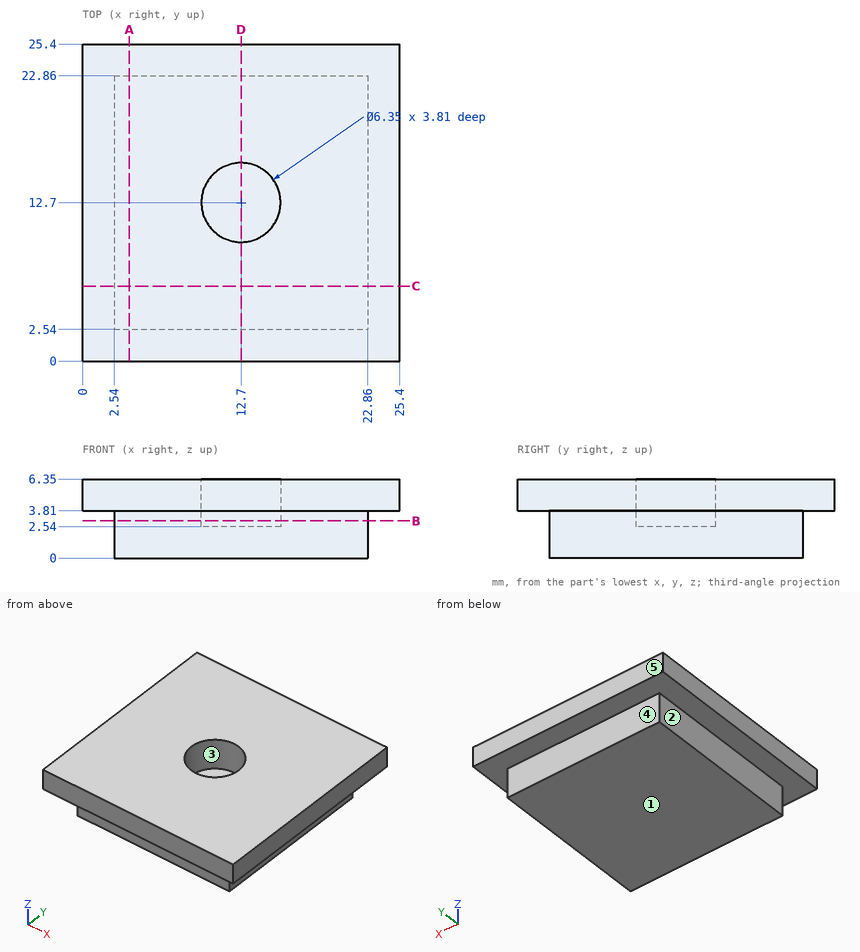
Source: three-view drawing plus pictorial views. Frame: mm from the lowest corner of the part. A direction names the side the tool comes from. Round coordinates to 2 decimals unless told otherwise and drop trailing zeros. Order: outer loops, then holes, each group sorted by start corner. A loop starts at its lowest first (then second) coordinate and runs counter-clockwise, first axis right, second up. Notation, with made-up numbers: (13.5, 30.25) - (23.5, 30.25) arc R36 cw to (23.5, 65.25) - close; hole circle Ø11 at (-35, -36.75). An arc over 180 degrees is marked (long way). Write each question's results on one line, items separated by ' | '.
Item 1: Section B-B, the plane z = 3. Return the cut outline in (x, y) (3 decimals), and give its area (3 significant figures).
Completed:
outline: (2.54, 2.54) - (22.86, 2.54) - (22.86, 22.86) - (2.54, 22.86) - close; hole circle Ø6.35 at (12.7, 12.7) | area: 381 mm^2
Item 2: Section A-A, the plane x = 3.75. Return the cut outline in (y, z).
Completed:
outline: (0, 3.81) - (2.54, 3.81) - (2.54, 0) - (22.86, 0) - (22.86, 3.81) - (25.4, 3.81) - (25.4, 6.35) - (0, 6.35) - close
Item 3: First-contact query: pin 1 Ø5 at (x, y) = (12.7, 12.7) entering from +Z; pin 2 Ø3 at (y, z) = (10.5, 1.5) entering from -X; pin 3 Ø3 at (x, z) = (13, 1.5) entering from -Y. Flat tips, straight axial feed; report the tip coordinate or a pass-through.
Completed:
pin 1: z = 2.54 | pin 2: x = 2.54 | pin 3: y = 2.54
Item 4: Mould query, pull axis X, two halves, no side actions, for the marked faces 1, 2 and 3. Classes: pulls with the +X half, pulls with the -X half, needs draft (parallel to the pull), parting line crosses it, or undercut.
Completed:
face 1: needs draft | face 2: pulls with the -X half | face 3: undercut
Item 5: Section D-D, the plane x = 12.7. Return the cut outline in (y, z) (3 decimals).
Completed:
outline: (0, 3.81) - (2.54, 3.81) - (2.54, 0) - (22.86, 0) - (22.86, 3.81) - (25.4, 3.81) - (25.4, 6.35) - (15.875, 6.35) - (15.875, 2.54) - (9.525, 2.54) - (9.525, 6.35) - (0, 6.35) - close
Item 6: Reachability of the marked faces 4 and 5 from +Z, -Z, +X, -X, +Y, -Y: full face, straight path, thin tool, end or side. Return the list, or none.
Completed:
face 4: -Z, +X, -X, +Y | face 5: +Z, -Z, +X, -X, +Y
Item 7: Material intervals for line 1 along Y through (x, z) = (12.7, 3.7) (3 decimals); line 2 along Y through (x, z) = (12.7, 3.95) (3 decimals); line 3 along X through (y, z) = (21.75, 1.75), sorted ascending. Write a range as [from, to].
Completed:
line 1: [2.54, 9.525], [15.875, 22.86] | line 2: [0, 9.525], [15.875, 25.4] | line 3: [2.54, 22.86]
